```python
from build123d import *

# Parameters (mm, degrees)
F0_W     = 85.4
F0_H     = 31.4
F0_W_2   = 2.6
F0_H_2   = 5.8
F0_R     = 2
F0_W_3   = 55.4
F0_H_3   = 25.4
F1_DEPTH = 4
F2_W     = 13.854876
F2_H     = 31.4
F2_W_2   = 2.6
F2_H_2   = 5.8
F2_R     = 2
F3_DEPTH = 4
F4_R     = 1.6
F5_DEPTH = 25
F6_SIZE  = 3


with BuildPart() as f1:
    # F0 (on Front) → F1 (new body)
    with BuildSketch(Plane.XZ):
        Rectangle(F0_W, F0_H)
        with Locations((-35.4, -6.336361)):
            Rectangle(F0_W_2, F0_H_2, mode=Mode.SUBTRACT)
        with Locations((-35.2, 8.7)):
            Circle(F0_R, mode=Mode.SUBTRACT)
        Rectangle(F0_W_3, F0_H_3, mode=Mode.SUBTRACT)
        with Locations((35.2, 0)):
            Circle(F0_R, mode=Mode.SUBTRACT)
    extrude(amount=F1_DEPTH)

    # F2 (on face) → F3 (join)
    with BuildSketch(Plane(origin=(0, 0, 0), x_dir=(-1, 0, 0), z_dir=(0, 1, 0))):
        with Locations((35.772562, 0)):
            Rectangle(F2_W, F2_H)
        with Locations((35.4, -6.336361)):
            Rectangle(F2_W_2, F2_H_2, mode=Mode.SUBTRACT)
        with Locations((35.2, 8.7)):
            Circle(F2_R, mode=Mode.SUBTRACT)
    extrude(amount=F3_DEPTH)

    # F4 (on face) → F5 (cut)
    with BuildSketch(Plane(origin=(-42.7, 0, 0), x_dir=(0, -1, 0), z_dir=(-1, 0, 0))):
        with Locations((0, -6.336361)):
            Circle(F4_R)
    extrude(amount=-F5_DEPTH, mode=Mode.SUBTRACT)

    # F6
    f6_edges = [f1.edges().sort_by_distance(p)[0] for p in [
        (-33.2, 4, 8.7),
        (33.2, 0, 0),
    ]]
    chamfer(f6_edges, length=F6_SIZE)


solid = f1.part
```
Design review of the part built by this model. Coordinates are the model's own, in mm. A direction names the side the tool comes from. Round coordinates to 2 decimals unless told otherwise and drop trailing zeros. Order: outer loops, then holes, each group sorted by start corner. A loop starts at its lowest first (then second) coordinate and runs counter-clockwise, first axis right, second up. Notation, with made-up numbers: M 6.5,64 L 17.5,64 A21 cw 17.5,84 Z; hole C -27.5,-31.75 d8. An arc over 180 degrees is marked long. Put each result on its own line as item: value.
Q1. To check wall thickness, follow line 1 (Z direction, x = -35.2, y = 0.85); line 2 (X direction, y = 1, z = -8); line 3 (Z direction, x = 3.5, y = -0.25). State the ranges of each line that lie inside material, in increasing order.
Reported:
line 1: -15.7 to -9.24, -3.44 to 6.7, 10.7 to 15.7
line 2: -42.7 to -36.7, -34.1 to -28.85
line 3: -15.7 to -12.7, 12.7 to 15.7
Q2. Consider section A-A (z = -10). State the section outline as (x, y) points.
Reported:
outline: M -42.7,-4 L -27.7,-4 L -27.7,0 L -28.85,0 L -28.85,4 L -42.7,4 Z; M 27.7,-4 L 42.7,-4 L 42.7,0 L 27.7,0 Z
Q3. Consider section D-D (x = -35.2). State the section outline as (y, z) points.
Reported:
outline: M -4,-15.7 L 4,-15.7 L 4,-9.24 L -4,-9.24 Z; M -4,-3.44 L 4,-3.44 L 4,3.7 L 1,6.7 L -4,6.7 Z; M -4,10.7 L 1,10.7 L 4,13.7 L 4,15.7 L -4,15.7 Z
Q4. Consider section C-C (z = 8.7). State the section outline as (x, y) points, and give its area (3 significant figures).
Reported:
outline: M -42.7,-4 L -37.2,-4 L -37.2,1 L -40.2,4 L -42.7,4 Z; M -33.2,-4 L -27.7,-4 L -27.7,0 L -28.85,0 L -28.85,4 L -30.2,4 L -33.2,1 Z; M 27.7,-4 L 42.7,-4 L 42.7,0 L 27.7,0 Z
area: 134 mm²
Q5. Consider section B-B (x = -15.5). State the section outline as (y, z) points, and give its area (3 significant figures).
Reported:
outline: M -4,-15.7 L 0,-15.7 L 0,-12.7 L -4,-12.7 Z; M -4,12.7 L 0,12.7 L 0,15.7 L -4,15.7 Z
area: 24.0 mm²
Q6. Machinability: for faces 5 (the face through (-35, 0, -3.436)), 6 (the face through (-28.845, 2, 0)), 7 (the face through (-36, 4, 0)), which of the approach directions +Z, -Z, +X, -X, +Y, -Y give a long, thin tool a straight path to every point of the face, cutting with its end or side? Answer none if there is none.
Reported:
face 5: +Y, -Y
face 6: +Z, -Z, +X, +Y
face 7: +Z, -Z, +X, -X, +Y
Q7. Insertion check: pin 1 Ø5 at (x, z) = (35.2, 0) entering from +Y. The pin has a flat end and moves straight along its axis. Give the tip position at first contact, or say it passes through.
Reported:
pin 1: y = -2.5
Q8. Draft analysis for pull direction Y (two halves, no side actions). For faces 1 (the face through (-1, -4, -14)), 2 (the face through (-35, 0, -9.236)), 3 (the face through (-39.74, 0.21, -4.75)), 4 (the face through (-30.945, -1.526, -5.856)), state which applies: released by +Y, released by -Y, zero draft, split by the parting line, or undercut.
Reported:
face 1: released by -Y
face 2: zero draft
face 3: undercut
face 4: undercut
